Check sheet for the modelled part. Datum: model origin and axes. Units: mm. A direction names the side the tool comes from. Give positions to 0.01 mm unless a question says otherwise; leave off trailing zeros. Order: outer loops, then holes, each group sorted by start corner. A loop starts at its lowest first (then second) coordinate and runs counter-clockwise, first axis right, second up.
```python
from build123d import *

# Parameters (mm, degrees)
SKICA1_W                      = 45
SKICA1_H                      = 45
SKICA1_W_2                    = 41
SKICA1_H_2                    = 41
P_IDAT_VYSUNUT_M1_DEPTH       = 20
ODEBRAT_VYSUNUT_M1_REACH      = 68.708
SKICA2_W                      = 15
SKICA2_H                      = 20
ODEBRAT_VYSUNUT_M2_DEPTH      = 67.708320321
ODEBRAT_VYSUNUT_M2_DEPTH_BACK = 67.708320321


with BuildPart() as part:
    # Skica1 → Přidat vysunutím1 (new body)
    with BuildSketch(Plane(origin=(0, 0, 0), x_dir=(1, 0, 0), z_dir=(0, 1, 0))):
        with Locations((22.5, -22.5)):
            Rectangle(SKICA1_W, SKICA1_H)
        with Locations((22.5, -22.5)):
            Rectangle(SKICA1_W_2, SKICA1_H_2, mode=Mode.SUBTRACT)
    extrude(amount=P_IDAT_VYSUNUT_M1_DEPTH)

    # Skica2 → Odebrat vysunutím1 (cut, up to next)
    with BuildSketch(Plane.XY.offset(45), mode=Mode.PRIVATE) as odebrat_vysunut_m1_sk1:
        with Locations((22.5, 10)):
            Rectangle(SKICA2_W, SKICA2_H)
    odebrat_vysunut_m1_tool1 = extrude(odebrat_vysunut_m1_sk1.sketch, amount=-ODEBRAT_VYSUNUT_M1_REACH, mode=Mode.PRIVATE) & part.part
    add(odebrat_vysunut_m1_tool1.solids().sort_by_distance((22.5, 10, 45))[0], mode=Mode.SUBTRACT)

    # Skica3 → Odebrat vysunutím2 (cut, two sides: drawn at the far end of the back side and taken through both)
    with BuildSketch(Plane.ZY.offset(-ODEBRAT_VYSUNUT_M2_DEPTH_BACK)):
        with BuildLine():
            ThreePointArc((25, 14.5), (24.267766953, 16.267766953), (22.5, 17))
            Line((22.5, 17), (22.5, 14.5))
            Line((22.5, 14.5), (25, 14.5))
        make_face()
        with BuildLine():
            Line((22.5, 14.5), (22.5, 17))
            ThreePointArc((22.5, 17), (20.732233047, 16.267766953), (20, 14.5))
            Line((20, 14.5), (22.5, 14.5))
        make_face()
        with BuildLine():
            Line((25, 14.5), (22.5, 14.5))
            Line((22.5, 14.5), (22.5, 12))
            ThreePointArc((22.5, 12), (24.267766953, 12.732233047), (25, 14.5))
        make_face()
        with BuildLine():
            Line((22.5, 12), (22.5, 14.5))
            Line((22.5, 14.5), (20, 14.5))
            ThreePointArc((20, 14.5), (20.732233047, 12.732233047), (22.5, 12))
        make_face()
        with BuildLine():
            Line((30.5, 20), (22.5, 20))
            Line((22.5, 20), (22.5, 17))
            ThreePointArc((22.5, 17), (24.267766953, 16.267766953), (25, 14.5))
            Line((25, 14.5), (30.5, 20))
        make_face()
        with BuildLine():
            Line((22.5, 17), (22.5, 20))
            Line((22.5, 20), (14.5, 20))
            Line((14.5, 20), (20, 14.5))
            ThreePointArc((20, 14.5), (20.732233047, 16.267766953), (22.5, 17))
        make_face()
    extrude(amount=ODEBRAT_VYSUNUT_M2_DEPTH + ODEBRAT_VYSUNUT_M2_DEPTH_BACK, mode=Mode.SUBTRACT)


solid = part.part
```
(1) Go/stop test with a flat-tipped pin: P1, Ø10, axis at x = 23.5, y = 6.5, coming from the +Z side. Record where the tip stops, or that it passes through.
(2) Sectioned sample at D-D (y = 2.5). Enter the section's corners in (x, z).
(3) Sectioned sample at A-A (y = 18.25). Enter the section's corners in (x, z).
(4) Tool access check on faces 1 (the face through (22, 0, 1)), 2 (the face through (30, 10, 44)), 3 (the face through (44, 17.2, 27.7)), 4 (the face through (36, 10, 43)). Record the directions out of +Z, -Z, +X, -X, +Y, -Y that give a thin tool (end or side, any length) a straight path to the whole face; none if there is none.
(5) Sectioned sample at C-C (z = 8). Enter the section's corners in (x, y).
(6) Sectioned sample at B-B (x = 32.5). Enter the section's corners in (y, z), plus the area to 3 significant figures.
(7) Release check for a two-part mould opening along X. For faces 5 (the face through (45, 10, 23)), 6 (the face through (43, 10, 23)), 7 (the face through (7, 10, 45)) record: released by +X, released by -X, zero draft, split by the parting line, or undercut.
(8) Thickness scan on L1, parallel to X at y = 7.75, z = 5; L2, parallel to Z at x = 20, y = 5. Record the ranges inside material, lowest first.
Values follow:
1. P1: stops at z = 2
2. outline: (0, 0) - (45, 0) - (45, 45) - (30, 45) - (30, 43) - (43, 43) - (43, 2) - (2, 2) - (2, 43) - (15, 43) - (15, 45) - (0, 45) - close
3. outline: (0, 0) - (45, 0) - (45, 16.25) - (43, 16.25) - (43, 2) - (2, 2) - (2, 16.25) - (0, 16.25) - close; (0, 28.75) - (2, 28.75) - (2, 43) - (15, 43) - (15, 45) - (0, 45) - close; (30, 43) - (43, 43) - (43, 28.75) - (45, 28.75) - (45, 45) - (30, 45) - close
4. face 1: +Z, -Z, +X, -X, -Y
4. face 2: +Z, +Y, -Y
4. face 3: +X, -X, +Y
4. face 4: +Y, -Y
5. outline: (0, 0) - (2, 0) - (2, 20) - (0, 20) - close; (43, 0) - (45, 0) - (45, 20) - (43, 20) - close
6. outline: (0, 0) - (20, 0) - (20, 2) - (0, 2) - close; (0, 43) - (20, 43) - (20, 45) - (0, 45) - close
6. area: 80.0 mm2
7. face 5: released by +X
7. face 6: undercut
7. face 7: zero draft
8. L1: x = 0 to 2, 43 to 45
8. L2: z = 0 to 2
